Read the model definition and answer for the solid it produces. Units are mm, in the model's axes. Face numbers are marked on the shaded views. A direction names the side the tool comes from. Coordinates: 2 decimals unless noted, no trailing zeros. Loops run counter-clockwise (first coordinate to the right, second up) from the corner with the lowest first, then second, coordinate; pieces in that order, holes last.
Q1. Section A-A (y = -17.5) is taken. Give the vertices of the cut face in (x, z).
Q2. Section B-B (z = -79.5) is taken. Give the vertices of the cut face in (x, y), then the cut area to 3 significant figures.
Q3. Which of the six approach directions +Z, -Z, +X, -X, +Y, -Y give full straight-line access (tool end or side, diameter ignored) to the marked faces 1 and 2?
Q4. Section C-C (x = 58) is taken. Give the vertices of the cut face in (y, z).
Q5. Straight lines are drawn through the part: line 1 (X direction, y = -17, z = -79); line 2 (Z direction, x = 30.5, y = -5); line 3 (X direction, y = -21, z = -70.5). For each, find the intervals that lie inside material, in ascending order.
Q6. Flat-ended cylindrical pins translate along their axes: P1, Ø2, axis at y = -13.5, z = -19.5, coming from the +X side; P2, Ø3, axis at x = 35, y = -18.5, coming from the -Z side; P3, Ø6.5, axis at x = 96.5, y = -13, coming from the -Z side. Find the tip coordinate at first contact, or state that the pin passes through.
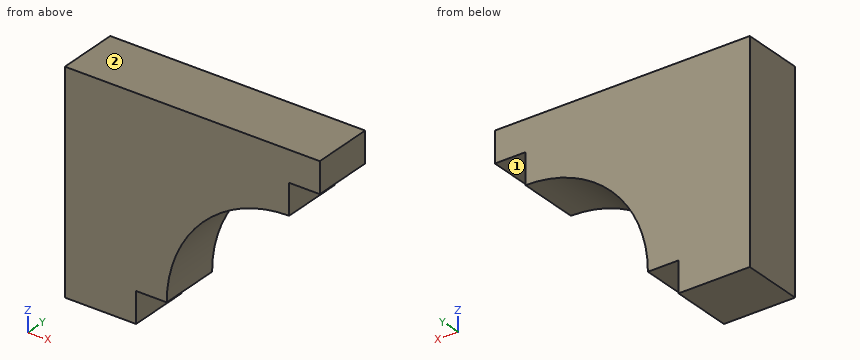
from build123d import *

# Parameters (mm, degrees)
F1_DEPTH = 25.4


with BuildPart() as f1:
    # F0 (on Front) → F1 (new body)
    with BuildSketch(Plane.XZ):
        with BuildLine():
            Line((105.758528, 0), (0, 0))
            Line((0, 0), (0, -88.9))
            Line((0, -88.9), (29.558528, -88.9))
            Line((29.558528, -88.9), (29.558528, -76.2))
            Line((29.558528, -76.2), (42.258528, -76.2))
            ThreePointArc((42.258528, -76.2), (57.137504, -40.278976), (93.058528, -25.4))
            Line((93.058528, -25.4), (93.058528, -12.7))
            Line((93.058528, -12.7), (105.758528, -12.7))
            Line((105.758528, -12.7), (105.758528, 0))
        make_face()
    extrude(amount=F1_DEPTH)


solid = f1.part
Numbers:
1. outline: (0, -88.9) - (29.56, -88.9) - (29.56, -76.2) - (42.26, -76.2) arc R50.8 cw to (93.06, -25.4) - (93.06, -12.7) - (105.76, -12.7) - (105.76, 0) - (0, 0) - close
2. outline: (0, -25.4) - (29.56, -25.4) - (29.56, 0) - (0, 0) - close
2. area: 751 mm2
3. face 1: -Z, +X, +Y, -Y
3. face 2: +Z, +X, -X, +Y, -Y
4. outline: (-25.4, -39.44) - (0, -39.44) - (0, 0) - (-25.4, 0) - close
5. line 1: x = 0 to 29.56
5. line 2: z = -76.2 to 0
5. line 3: x = 0 to 42.58
6. P1: stops at x = 93.06
6. P2: stops at z = -76.2
6. P3: stops at z = -12.7
